Design review of the part built by this model. Coordinates are the model's own, in mm. A direction names the side the tool comes from. Coordinates: 2 decimals unless noted, no trailing zeros. Loops run counter-clockwise (first coordinate to the right, second up) from the corner with the lowest first, then second, coordinate; pieces in that order, holes last.
from build123d import *

# Parameters (mm, degrees)
F0_W          = 10
F0_H          = 16
F1_DEPTH      = 1.5
F2_W          = 4
F2_H          = 4
F3_DEPTH      = 2.5
F3_DEPTH_BACK = 1.5
F4_R          = 1.5
F5_R          = 1.25
F6_DEPTH      = 8.001
F8_DEPTH      = 3
F10_R         = 1
F9_W          = 9
F9_H          = 1.5
F11_DEPTH     = 11.001
F12_W         = 4
F12_H         = 1
F13_DEPTH     = 1.5


with BuildPart() as f1:
    # F0 (on Front) → F1 (new body)
    with BuildSketch(Plane.XZ):
        with Locations((-5, 8)):
            Rectangle(F0_W, F0_H)
    extrude(amount=F1_DEPTH)

    # F2 (on face) → F3 (join, two sides)
    with BuildSketch(Plane.XZ.offset(1.5)) as f3_sk:
        with Locations((-6, -1.5)):
            Rectangle(F2_W, F2_H)
    extrude(amount=F3_DEPTH)
    extrude(f3_sk.sketch, amount=-F3_DEPTH_BACK)

    # F4
    f4_edges = [f1.edges().sort_by_distance(p)[0] for p in [
        (-6, 0, -3.5),
        (-6, -4, -3.5),
        (-6, -4, 0.5),
    ]]
    fillet(f4_edges, radius=F4_R)

    # F5 (on face) → F6 (cut, through all)
    with BuildSketch(Plane(origin=(-8, 0, 0), x_dir=(0, -1, 0), z_dir=(-1, 0, 0))):
        with Locations((2, -1.5)):
            Circle(F5_R)
    extrude(amount=-F6_DEPTH, mode=Mode.SUBTRACT)

    # F7 (on face) → F8 (join)
    with BuildSketch(Plane.XZ.offset(1.5)):
        Polygon((-10, 16), (-10, 5), (-7, 5), (-7, 14.5), (0, 14.5), (0, 16), align=None)
    extrude(amount=F8_DEPTH)

    # F10
    f10_edges = [f1.edges().sort_by_distance(p)[0] for p in [
        (-10, -4.5, 10.5),
    ]]
    fillet(f10_edges, radius=F10_R)

    # F9 (on face) → F11 (cut, through all)
    with BuildSketch(Plane.XY.offset(16)):
        with Locations((-4.5, -2.25)):
            Rectangle(F9_W, F9_H)
    extrude(amount=-F11_DEPTH, mode=Mode.SUBTRACT)

    # F12 (on face) → F13 (cut)
    with BuildSketch(Plane.XZ.offset(1.5)):
        with Locations((-2, 0.5)):
            Rectangle(F12_W, F12_H)
    extrude(amount=-F13_DEPTH, mode=Mode.SUBTRACT)

    # F14: F1 across plane


with BuildPart() as f1_1:
    add(f1.part)
    add(f1.part.mirror(Plane.YZ))


solid = f1_1.part
Q1. Take a section at B-B, the plane y = -2. Write out the cut boundary in (x, z).
Q2. Take a section at D-D, the plane z = -1.5. Write out the cut boundary in (x, y).
Q3. Take a section at C-C, the plane x = 3.75. Write out the cut boundary in (y, z), then the cut area to 4 significant figures.
Q4. Take a section at A-A, the plane x = -5.5. Write out the cut boundary in (y, z).
Q5. For line 1 (Z direction, x = 5.8, y = -2); line 2 (X direction, y = -1.45, z = -0.25); line 3 (X direction, y = -2.85, z = 6.5), list the stretches that pass through material, from the lowest coordinate up.
Q6. The part is to be moulded in two halves that separate along Z. For faces 1 (the cylindrical face through (6.028, -3.155, -1.979)), 2 (the cylindrical face through (-5.97, -3.55, -3.07)), 3 (the flat face through (0, -4, 14.5)), 4 (the flat face through (0, 0, 7)), say which applies: pulls with the +Z half, pulls with the -Z half, needs draft (parallel to the pull), parting line crosses it, or undercut.
Q7. Machinability: for faces 5 (the cylindrical face through (-5.97, -3.57, 0.05)), 6 (the flat face through (6, -4, -1.5)), 7 (the flat face through (6, -2, 0.5)), 8 (the flat face through (4, -2, 0)), which of the approach directions +Z, -Z, +X, -X, +Y, -Y give a long, thin tool a straight path to every point of the face, cutting with its end or side? Answer none if there is none.
Q8. Clearance check with flat-ended pins moving along their axes: pin 1 Ø0.8 at (x, y) = (-9, -1) entering from -Z; pin 2 Ø2 at (y, z) = (-2, -1.5) entering from +X; pin 3 Ø1.5 at (x, y) = (-9, -3.5) entering from -Z; pin 4 Ø0.8 at (x, z) = (6, -1.5) entering from -Y. State where each tip first meets the part, or that it passes through.
Entries:
1. outline: (-10, 5) - (-9, 5) - (-9, 16) - (-10, 16) - close; (-8, -3.5) - (-4, -3.5) - (-4, -2.75) - (-8, -2.75) - close; (-8, -0.25) - (-4, -0.25) - (-4, 0.5) - (-8, 0.5) - close; (4, -3.5) - (8, -3.5) - (8, -2.75) - (4, -2.75) - close; (4, -0.25) - (8, -0.25) - (8, 0.5) - (4, 0.5) - close; (9, 5) - (10, 5) - (10, 16) - (9, 16) - close
2. outline: (-8, -4) - (-4, -4) - (-4, -3.25) - (-8, -3.25) - close; (-8, -0.75) - (-4, -0.75) - (-4, 0) - (-8, 0) - close; (4, -4) - (8, -4) - (8, -3.25) - (4, -3.25) - close; (4, -0.75) - (8, -0.75) - (8, 0) - (4, 0) - close
3. outline: (-4.5, 14.5) - (-3, 14.5) - (-3, 16) - (-4.5, 16) - close; (-1.5, 1) - (0, 1) - (0, 16) - (-1.5, 16) - close
3. area: 24.75 mm2
4. outline: (-4.5, 14.5) - (-3, 14.5) - (-3, 16) - (-4.5, 16) - close; (-4, -2) arc R1.5 ccw to (-2.5, -3.5) - (-1.5, -3.5) arc R1.5 ccw to (0, -2) - (0, 16) - (-1.5, 16) - (-1.5, 0.5) - (-2.5, 0.5) arc R1.5 ccw to (-4, -1) - close; hole circle Ø2.5 at (-2, -1.5)
5. line 1: z = -3.5 to -2.75, -0.25 to 0.5
5. line 2: x = -8 to -4, 4 to 8
5. line 3: x = -10 to -9, 9 to 10
6. face 1: undercut
6. face 2: pulls with the -Z half
6. face 3: undercut
6. face 4: needs draft
7. face 5: +X, -X, -Y
7. face 6: -Z, +X, -X, -Y
7. face 7: +Z, +X, -X, -Y
7. face 8: -Z, +Y, -Y
8. pin 1: stops at z = 0
8. pin 2: passes through
8. pin 3: stops at z = 5
8. pin 4: stops at y = -4
